Can you work these out from the model? Positions are in its coordinate system, mm. A direction names the side the tool comes from. Coordinates: 2 decimals unless noted, no trailing zeros. Write each loop counter-clockwise with the first axis right and the second up, starting at its lowest first coordinate (ties: lowest second). Pieces come first, ordered by that corner, then holes. Notation, with made-up numbers: (89, 79.25) -> (116, 79.25) arc R28 cw to (116, 112.25) -> close; hole circle Ø9 at (10.25, 81). An arc over 180 degrees is marked (long way). Use one line per item in the form item = value.
```python
from build123d import *


with BuildPart() as f1:
    # F0 (on Front) → F1 (revolve)
    with BuildSketch(Plane.XZ):
        Polygon((-3.403124, 3.403124), (0, 0), (0, 1.5), (-9.545942, 11.045942), (-9.545942, 29.580235), (-10.686858, 28.606423), (-10.606602, 10.606602), align=None)
        Polygon((0, -5), (0, 0), (-3.403124, 3.403124), (-0.361914, -5), align=None)
        Polygon((0, -6), (0, -5), (-0.361914, -5), align=None)
        Polygon((0, -6), (-0.361914, -5), (-1, -5), (-1, -6), align=None)
        Polygon((0, -9), (0, -6), (-1, -6), align=None)
        Polygon((1.999995, -9.004474), (0, -6), (0, -9), align=None)
        Polygon((1.999995, -9.004474), (0, -9), (1.993284, -12.004467), align=None)
    revolve(axis=Axis((2.5, 0, 17.566036), (0, 0, 1)))


solid = f1.part
```
Q1. If I drill on line 1 (Y direction, x = 2.5, z = -3.5); line 2 (Y direction, x = 2.5, z = -1); line 3 (X direction, y = 0, z = 23.75), over which ranges is the centre line in solid material (lowest first)? Write a range as from..to.
Return value:
line_1 = -3.4..-2.5, 2.5..3.4
line_2 = -4.31..-2.5, 2.5..4.31
line_3 = -10.67..-9.55, 14.55..15.67
Q2. For faces 1 (the cylindrical face through (0.115, -0.751, -2.198)), 2 (the flat face through (3, 3, -5)), 3 (the conical face through (5.35, 12.834, 19.481)), which set-ups out of +Z, -Z, +X, -X, +Y, -Y let a thin tool reach every point of the face, with its end or its side?
Return value:
face_1 = +Z
face_2 = none
face_3 = -Z
Q3. Will these pins go through, and if not, where does the flat tip stop? pin 1 (1.5 mm diameter, centred on y = -6.5, z = 12, fed in from -X); pin 2 (8 mm diameter, centred on y = 0.5, z = -5, fed in from -X); pin 3 (4 mm diameter, centred on x = -7.5, y = -3.5, fed in from -Z).
Return value:
pin_1 = -9.28
pin_2 = -1.8
pin_3 = 6.09
Q4. Suppose I cut it at B-B (z = -4). Write out the boundary of the cut face in (x, y).
Return value:
outline = circle Ø6.45 at (2.5, 0); hole circle Ø5 at (2.5, 0)
Q5. Suppose I cut it at A-A (z = 10). Write out the boundary of the cut face in (x, y).
Return value:
outline = circle Ø25 at (2.5, 0); hole circle Ø22 at (2.5, 0)
Q6. Thinking about a two-plate mould opening in X: for faces 4 (the conical face through (3.003, -0.022, -10.483)), 5 (the conical face through (1.5, -0.31, -11.19)), which applies, released by +X, released by -X, zero draft, split by the parting line, or undercut?
Return value:
face_4 = undercut
face_5 = split by the parting line
